from build123d import *

# Parameters (mm, degrees)
BOSS_EXTRUDE1_DEPTH = 1.5
SKETCH2_W           = 3
SKETCH2_H           = 10
BOSS_EXTRUDE2_DEPTH = 14
SKETCH3_W           = 10
SKETCH3_H           = 2
BOSS_EXTRUDE3_DEPTH = 12


with BuildPart() as part:
    # Sketch1 → Boss-Extrude1 (new body)
    with BuildSketch(Plane(origin=(0, 0, 0), x_dir=(1, 0, 0), z_dir=(0, 1, 0))):
        Polygon((-10.528994658, 3.760355235), (-10.528994658, 28.760355235), (-20.528994658, 28.760355235), (-20.528994658, -6.239644765), (17.471005342, -6.239644765), (17.471005342, 3.760355235), align=None)
    extrude(amount=BOSS_EXTRUDE1_DEPTH)

    # Sketch2 → Boss-Extrude2 (add)
    with BuildSketch(Plane.XZ):
        with Locations((15.971005342, 1.239644765)):
            Rectangle(SKETCH2_W, SKETCH2_H)
    extrude(amount=BOSS_EXTRUDE2_DEPTH)

    # Sketch3 → Boss-Extrude3 (add)
    with BuildSketch(Plane.ZY.offset(-14.471005342)):
        with Locations((1.239644765, -13)):
            Rectangle(SKETCH3_W, SKETCH3_H)
    extrude(amount=BOSS_EXTRUDE3_DEPTH)


solid = part.part
Could you check a few things on this model? Use its own coordinates, in mm. A direction names the side the tool comes from. Give positions to 0.01 mm unless a question says otherwise; leave off trailing zeros. Write each loop counter-clockwise with the first axis right and the second up, starting at its lowest first coordinate (ties: lowest second). Pieces come first, ordered by that corner, then holes. Notation, with made-up numbers: (75.25, 44) - (113.25, 44) arc R30 cw to (113.25, 75) - close; hole circle Ø4 at (-20.75, -5.75). An arc over 180 degrees is marked (long way). Use CSV: the item, a comma, the result in double quotes. Start each with the question number.
Item 1: I want a section at B-B, the plane y = -2.5. Please give me the cut outline in (x, z), then the cut area to 3 significant figures.
Item 2: I'm going to push flat-ended pins straight in: pin 1 (5 mm diameter, centred on y = -6, z = 1.5, fed in from -X); pin 2 (10.5 mm diameter, centred on x = -11.5, z = -8.5, fed in from -Y); pin 3 (0.8 mm diameter, centred on y = 0.5, z = -16.5, fed in from +X); pin 4 (6 mm diameter, centred on x = -6.5, z = -10.5, fed in from +Y). Where does each tip first touch, or does it pass through?
Item 3: I want a section at A-A, the plane z = -1. Please give me the cut outline in (x, y).
Item 4: For faces 4 (the face through (-10.529, 1, -16)), 5 (the face through (2.471, -13, 1)), 6 (the face through (9, -12, 1)), which set-ups out of +Z, -Z, +X, -X, +Y, -Y let a thin tool reach every point of the face, with its end or its side?
Item 5: If I drill on line 1 along Y through (x, z) = (9, 4); line 2 along X through (y, z) = (-9.25, 1.5); line 3 along X through (y, z) = (0.75, -16), over which ranges is the centre line in solid material (lowest first)?
Item 6: I want a section at C-C, the plane x = -16. Please give me the cut outline in (y, z), then the cut area to 3 significant figures.
Item 7: If we mould it in two halves opening along Y, with no side actions, what happens to faces 1 (the face through (-6, 1.5, 0)), 2 (the face through (14.471, -6, 1)), 3 (the face through (-15, 1, -28.76))? For each: pulls with the +Y half, pulls with the -Y half, needs draft (parallel to the pull), parting line crosses it, or undercut.
Findings:
1,outline,"(14.47, -3.76) - (17.47, -3.76) - (17.47, 6.24) - (14.47, 6.24) - close"
1,area,"30.0 mm2"
2,pin 1,"stops at x = 14.47"
2,pin 2,"stops at y = 0"
2,pin 3,"stops at x = -10.53"
2,pin 4,"passes through"
3,outline,"(-20.53, 0) - (14.47, 0) - (14.47, -12) - (2.47, -12) - (2.47, -14) - (17.47, -14) - (17.47, 1.5) - (-20.53, 1.5) - close"
4,face 4,"-Z, +X, +Y, -Y"
4,face 5,"+Z, -Z, -X, -Y"
4,face 6,"+Z, -Z, -X"
5,line 1,"y = -14 to -12, 0 to 1.5"
5,line 2,"x = 14.47 to 17.47"
5,line 3,"x = -20.53 to -10.53"
6,outline,"(0, -28.76) - (1.5, -28.76) - (1.5, 6.24) - (0, 6.24) - close"
6,area,"52.5 mm2"
7,face 1,"pulls with the +Y half"
7,face 2,"undercut"
7,face 3,"needs draft"
